Work out the finished part from the listing and answer in its coordinate system (mm). A direction names the side the tool comes from. Give positions to 0.01 mm unless a question says otherwise; leave off trailing zeros. Write each loop counter-clockwise with the first axis right and the second up, starting at its lowest first coordinate (ties: lowest second). Pieces come first, ordered by that corner, then holes. Notation, with made-up numbers: (-6, -18.5) -> (47, -18.5) arc R27 ccw to (47, 11.5) -> close; hole circle Ø11 at (4.5, 3). An arc over 180 degrees is marked (long way). Write item = value, one per line. Start each with the question number.
from build123d import *

# Parameters (mm, degrees)
BOSS_EXTRU_1_DEPTH      = 10
ESQUISSE2_W             = 5
ESQUISSE2_H             = 30
ENL_V_MAT_EXTRU_1_DEPTH = 62.64414003
ESQUISSE3_R             = 1.5
ENL_V_MAT_EXTRU_2_DEPTH = 63.967823601
ESQUISSE5_R             = 1.5
ENL_V_MAT_EXTRU_3_DEPTH = 63.967823601
ENL_V_MAT_EXTRU_4_DEPTH = 63.967823601
CONG_VARIABLE1_R        = 2
CONG_4_R                = 20


with BuildPart() as part:
    # Esquisse1 → Boss.-Extru.1 (new body)
    with BuildSketch(Plane.XY):
        with BuildLine():
            ThreePointArc((0, -35), (1.835599765, -46.978253407), (7.173927734, -57.857142857))
            ThreePointArc((7.173927734, -57.857142857), (14.134329624, -59.103259033), (15.380445801, -52.142857143))
            ThreePointArc((15.380445801, -52.142857143), (11.376699824, -43.983690055), (10, -35))
            Line((10, -35), (10, 0))
            Line((10, 0), (0, 0))
            Line((0, 0), (0, -35))
        make_face()
    extrude(amount=BOSS_EXTRU_1_DEPTH)

    # Esquisse2 → Enl_v. mat.-Extru.1 (cut, through all)
    with BuildSketch(Plane(origin=(10, 0, 0), x_dir=(0, 0, -1), z_dir=(1, 0, 0))):
        with Locations((-5, -15)):
            Rectangle(ESQUISSE2_W, ESQUISSE2_H)
    extrude(amount=-ENL_V_MAT_EXTRU_1_DEPTH, mode=Mode.SUBTRACT)

    # Esquisse3 → Enl_v. mat.-Extru.2 (cut, through all)
    with BuildSketch(Plane.XY.offset(10)):
        with Locations((5, -5)):
            Circle(ESQUISSE3_R)
    extrude(amount=-ENL_V_MAT_EXTRU_2_DEPTH, mode=Mode.SUBTRACT)

    # Esquisse5 → Enl_v. mat.-Extru.3 (cut, through all)
    with BuildSketch(Plane.XY.offset(10)):
        with Locations((5, -25)):
            Circle(ESQUISSE5_R)
    extrude(amount=-ENL_V_MAT_EXTRU_3_DEPTH, mode=Mode.SUBTRACT)

    # Esquisse6 → Enl_v. mat.-Extru.4 (cut, through all)
    with BuildSketch(Plane.XY.offset(10)):
        with BuildLine():
            Line((14.840420876, -58.507614957), (1.835599765, -46.978253407))
            ThreePointArc((1.835599765, -46.978253407), (4.090400233, -52.621028477), (7.173927734, -57.857142857))
            ThreePointArc((7.173927734, -57.857142857), (10.854475024, -59.982099435), (14.840420876, -58.507614957))
        make_face()
    extrude(amount=-ENL_V_MAT_EXTRU_4_DEPTH, mode=Mode.SUBTRACT)

    # Cong_ variable1
    cong_variable1_edges = [part.edges().sort_by_distance(p)[0] for p in [
        (14.840420876, -58.507614957, 5),
    ]]
    fillet(cong_variable1_edges, radius=CONG_VARIABLE1_R)

    # Cong_4
    cong_4_edges = [part.edges().sort_by_distance(p)[0] for p in [
        (1.835599765, -46.978253407, 5),
    ]]
    fillet(cong_4_edges, radius=CONG_4_R)


solid = part.part
(1) A cutting plane is placed at A-A, the plane y = -5. Write down the section's boundary in (x, z), then the cut area to 3 significant figures.
(2) A cutting plane is placed at B-B, the plane z = 1.25. Write down the section's boundary in (x, y).
(3) For faces 1 (the flat face through (5, -15, 7.5)), 2 (the flat face through (10, -18, 2)), 3 (the cylindrical face through (2.156, -45.332, 4.93)), determine the directions among +Z, -Z, +X, -X, +Y, -Y from which every point of the face is accessible in a straight line to the end or side of a thin tool.
(4) A cutting plane is placed at D-D, the plane x = 2.25. Write down the section's boundary in (y, z), then the cut area to 3 significant figures.
(5) Find the intervals of material crossed by line 1 along Z through (x, y) = (6.75, -9); line 2 along Y through (x, z) = (5, 1.7); line 3 along X through (y, z) = (-31.5, 2.25), in increasing order.
(6) Determine the mould class of faces 4 (the flat face through (6, -28, 0)), 5 (the flat face through (5, -15, 2.5)), 6 (the cylindrical face through (14.953, -57.196, 4.93)) for opening direction Z: pulls with the +Z half, pulls with the -Z half, needs draft (parallel to the pull), parting line crosses it, or undercut.
(7) Each of these flat-tipped pins is pushed along its axis until it touches: pin 1 (4 mm diameter, centred on x = 3, z = 6, fed in from -Y); pin 2 (6 mm diameter, centred on x = 4.5, z = 4, fed in from -Y); pin 3 (5 mm diameter, centred on x = 5, y = -25, fed in from -Z); pin 4 (2.5 mm diameter, centred on x = 6, z = 4.5, fed in from +Y). Where does it stop, or does it pass through?
(8) A cutting plane is placed at C-C, the plane x = 6. Write down the section's boundary in (y, z), then the cut area to 3 significant figures.
Results list:
q1.outline = (0, 0) -> (3.5, 0) -> (3.5, 2.5) -> (0, 2.5) -> close; (0, 7.5) -> (3.5, 7.5) -> (3.5, 10) -> (0, 10) -> close; (6.5, 0) -> (10, 0) -> (10, 2.5) -> (6.5, 2.5) -> close; (6.5, 7.5) -> (10, 7.5) -> (10, 10) -> (6.5, 10) -> close
q1.area = 35.0 mm²
q2.outline = (0, -35) arc R40 ccw to (0.1, -37.79) arc R20 ccw to (6.78, -51.36) -> (12.93, -56.82) arc R2 ccw to (16.25, -55.53) arc R5 ccw to (15.38, -52.14) arc R30 cw to (10, -35) -> (10, 0) -> (0, 0) -> close; hole circle Ø3 at (5, -25); hole circle Ø3 at (5, -5)
q3.face_1 = +X, -X, +Y
q3.face_2 = +Z, -Z, +X, +Y
q3.face_3 = +Z, -Z, -X, -Y
q4.outline = (-45.52, 0) -> (0, 0) -> (0, 2.5) -> (-30, 2.5) -> (-30, 7.5) -> (0, 7.5) -> (0, 10) -> (-45.52, 10) -> close
q4.area = 305 mm²
q5.line_1 = 0 to 2.5, 7.5 to 10
q5.line_2 = -49.57 to -26.5, -23.5 to -6.5, -3.5 to 0
q5.line_3 = 0 to 10
q6.face_4 = pulls with the -Z half
q6.face_5 = undercut
q6.face_6 = needs draft
q7.pin_1 = -49.57
q7.pin_2 = -52
q7.pin_3 = 0
q7.pin_4 = -30
q8.outline = (-50.63, 0) -> (-26.12, 0) -> (-26.12, 2.5) -> (-30, 2.5) -> (-30, 7.5) -> (-26.12, 7.5) -> (-26.12, 10) -> (-50.63, 10) -> close; (-23.88, 0) -> (-6.12, 0) -> (-6.12, 2.5) -> (-23.88, 2.5) -> close; (-23.88, 7.5) -> (-6.12, 7.5) -> (-6.12, 10) -> (-23.88, 10) -> close; (-3.88, 0) -> (0, 0) -> (0, 2.5) -> (-3.88, 2.5) -> close; (-3.88, 7.5) -> (0, 7.5) -> (0, 10) -> (-3.88, 10) -> close
q8.area = 334 mm²
